Build history of the part. All positions in model axes, mm. Round coordinates to 2 decimals unless told otherwise and drop trailing zeros. Loops run counter-clockwise (first coordinate to the right, second up) from the corner with the lowest first, then second, coordinate; pieces in that order, holes last. Notation, with made-up numbers: (-30.75, 11.25) -> (-20.75, 11.25) arc R33 ccw to (-20.75, 40.25) -> close; hole circle Ø4 at (6, 13.25). An arc over 180 degrees is marked (long way). Put each result on its own line as item: value. Start each with the question number.
Item 1: Flat gauge pins, fed straight in: pin 1 Ø1.5 at (y, z) = (5, 6.5) entering from -X; pin 2 Ø6 at (x, y) = (14.5, 3.5) entering from -Z. Where does each tip first touch, or does it go through?
Item 2: Cut at A-A, the plane x = 44. List the corners of the cut face in (y, z), plus the area to 3 significant figures.
Item 3: Drill centre lines: probe 1 along X at (y, z) = (2.5, 7.5); probe 2 along X at (y, z) = (1, 5.5); probe 3 along X at (y, z) = (3.75, 3.75). Where is each one in solid material? Low to high. Write a range as [from, to].
```python
from build123d import *

# Parameters (mm, degrees)
SKETCH1_R           = 1
BOSS_EXTRUDE1_DEPTH = 8
CUT_EXTRUDE1_START  = -10
CUT_EXTRUDE1_DEPTH  = 10


with BuildPart() as part:
    # Sketch1 → Boss-Extrude1 (new body)
    with BuildSketch(Plane.XY):
        with BuildLine():
            Line((-4.413883096, 7.780619908), (48, 0))
            Line((48, 0), (58, 0))
            ThreePointArc((58, 0), (59.414213562, 0.585786438), (60, 2))
            Line((60, 2), (60, 11))
            ThreePointArc((60, 11), (59.414213562, 12.414213562), (58, 13))
            Line((58, 13), (-2, 13))
            ThreePointArc((-2, 13), (-3.042889965, 12.706569811), (-3.779764531, 11.912380521))
            Line((-3.779764531, 11.912380521), (-5.156928621, 9.22597091))
            ThreePointArc((-5.156928621, 9.22597091), (-5.156403682, 8.312567847), (-4.413883096, 7.780619908))
        make_face()
        with Locations((53.689231255, 9)):
            Circle(SKETCH1_R, mode=Mode.SUBTRACT)
    extrude(amount=BOSS_EXTRUDE1_DEPTH)

    # Sketch2 → Cut-Extrude1 (cut)
    with BuildSketch(Plane.XY.offset(8).offset(CUT_EXTRUDE1_START)):
        Polygon((-2.939974596, 7.561824407), (-0.965260048, 7.26868636), (-1.698752327, 9.125408347), align=None)
        with BuildLine():
            Line((-4.413883096, 7.780619908), (-3.685452086, 7.672487397))
            Line((-3.685452086, 7.672487397), (-4.418944365, 9.529209384))
            Line((-4.418944365, 9.529209384), (-5.231519115, 8.505598334))
            ThreePointArc((-5.231519115, 8.505598334), (-4.930484846, 8.021549823), (-4.413883096, 7.780619908))
        make_face()
        Polygon((-0.219982955, 7.158053119), (1.755132364, 6.864855579), (1.021491222, 8.72195439), align=None)
        Polygon((2.500209083, 6.754252082), (4.475324402, 6.461054542), (3.74168326, 8.318153353), align=None)
        Polygon((5.220200725, 6.350480793), (7.195716813, 6.057223761), (6.461926809, 7.914699396), align=None)
        Polygon((7.940392763, 5.946679757), (9.915908851, 5.653422725), (9.182118847, 7.510898359), align=None)
        Polygon((10.660384404, 5.542908468), (12.636301263, 5.249591943), (11.902362396, 7.107444402), align=None)
        Polygon((13.380576442, 5.139107432), (15.356493301, 4.845790907), (14.622554434, 6.703643365), align=None)
        Polygon((16.100568083, 4.735336143), (18.076885713, 4.441960126), (17.342797982, 6.300189408), align=None)
        Polygon((18.820760121, 4.331535107), (20.797077751, 4.038159089), (20.06299002, 5.896388371), align=None)
        Polygon((21.540751763, 3.927763818), (23.517470163, 3.634328308), (22.783233569, 5.492934414), align=None)
        Polygon((24.260943801, 3.523962782), (26.237662201, 3.230527271), (25.503425607, 5.089133377), align=None)
        Polygon((26.980935442, 3.120191493), (28.958054613, 2.82669649), (28.223669156, 4.68567942), align=None)
        Polygon((29.70112748, 2.716390456), (31.678246651, 2.422895453), (30.943861194, 4.281878383), align=None)
        Polygon((46.021678518, 0.293673481), (48, 0), (47.265167954, 1.860113401), align=None)
        Polygon((43.30148648, 0.697474518), (45.279807962, 0.403801037), (44.544975916, 2.263914437), align=None)
        Polygon((40.581494839, 1.101245806), (42.55941555, 0.807631818), (41.824732367, 2.667368395), align=None)
        Polygon((37.861302801, 1.505046843), (39.839223512, 1.211432854), (39.104540329, 3.071169432), align=None)
        Polygon((35.141311159, 1.908818131), (37.1188311, 1.615263636), (36.384296781, 3.474623389), align=None)
        Polygon((32.421119121, 2.312619168), (34.398639063, 2.019064672), (33.664104743, 3.878424426), align=None)
    extrude(amount=CUT_EXTRUDE1_DEPTH, mode=Mode.SUBTRACT)


solid = part.part
```
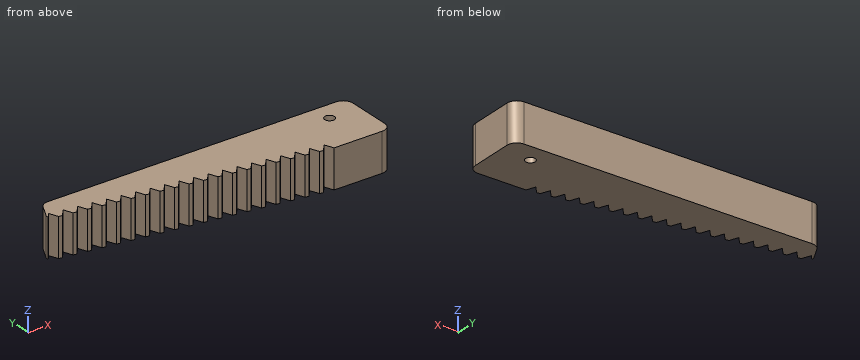
Reply:
1. pin 1: stops at x = 9.88
1. pin 2: stops at z = 0
2. outline: (1.58, 0) -> (13, 0) -> (13, 8) -> (1.58, 8) -> close
2. area: 91.4 mm^2
3. probe 1: x = [31.65, 32.57], [34.21, 35.61], [36.77, 38.65], [39.33, 41.69], [41.89, 60]
3. probe 2: x = [42.48, 43.54], [45.04, 46.58], [47.6, 59.73]
3. probe 3: x = [23.47, 24.44], [26.03, 27.48], [28.59, 30.52], [31.15, 33.56], [33.71, 60]
